Design review of the part built by this model. Coordinates are the model's own, in mm. Coordinates: 2 decimals unless noted, no trailing zeros. Write each loop counter-clockwise with the first axis right and the second up, starting at its lowest first coordinate (ties: lowest second). Pieces come first, ordered by that corner, then holes. Notation, with made-up numbers: M 60.25,-38.5 L 92.25,-38.5 A26 ccw 92.25,-21.5 Z; hole C -10.75,67.25 d7. An arc over 180 degrees is marked long. Write item = value, one per line.
```python
from build123d import *

# Parameters (mm, degrees)
BOSS_EXTRUDE1_DEPTH     = 5.5
CUT_EXTRUDE1_DEPTH      = 907.379197687
CUT_EXTRUDE1_DEPTH_BACK = 907.379197687
SKETCH2_R               = 1.6
SKETCH2_W               = 18
SKETCH2_H               = 13
SKETCH3_R               = 2.1
CUT_EXTRUDE2_DEPTH      = 907.379197687
SKETCH4_R               = 1.6
CUT_EXTRUDE3_DEPTH      = 907.379197687
SKETCH5_W               = 3.25
SKETCH5_H               = 9.45
SKETCH5_H_2             = 2.65
SKETCH5_W_2             = 1.25
SKETCH5_H_3             = 3.25
BOSS_EXTRUDE2_DEPTH     = 5.5


with BuildPart() as part:
    # Sketch1 → Boss-Extrude1 (new body)
    with BuildSketch(Plane.XY):
        Polygon((308.5, 78), (308.5, 50.625), (303, 50.625), (303, 42.125), (306.25, 42.125), (306.25, 40.5), (306.25, 38.875), (303, 38.875), (303, 30.375), (308.5, 30.375), (308.5, 3), (378, 3), (378, 8.5), (451.375, 8.5), (451.375, 17.95), (450.125, 17.95), (450.125, 20.6), (451.375, 20.6), (451.375, 23.25), (454.625, 23.25), (454.625, 20.6), (455.875, 20.6), (455.875, 17.95), (454.625, 17.95), (454.625, 8.5), (528, 8.5), (528, 3), (678, 3), (678, 8.5), (751.375, 8.5), (751.375, 17.95), (750.125, 17.95), (750.125, 20.6), (751.375, 20.6), (751.375, 23.25), (754.625, 23.25), (754.625, 20.6), (755.875, 20.6), (755.875, 17.95), (754.625, 17.95), (754.625, 8.5), (828, 8.5), (828, 3), (897.5, 3), (897.5, 30.375), (903, 30.375), (903, 38.875), (899.75, 38.875), (899.75, 40.5), (899.75, 42.125), (903, 42.125), (903, 50.625), (897.5, 50.625), (897.5, 78), align=None)
    extrude(amount=BOSS_EXTRUDE1_DEPTH)

    # Sketch2 → Cut-Extrude1 (cut, two sides: drawn at the far end of the back side and taken through both)
    with BuildSketch(Plane.XY.offset(5.5).offset(-CUT_EXTRUDE1_DEPTH_BACK)):
        with Locations((582.5, 40.5)):
            Circle(SKETCH2_R)
        with Locations((623.5, 40.5)):
            Circle(SKETCH2_R)
        with Locations((603, 40.5)):
            Rectangle(SKETCH2_W, SKETCH2_H)
    extrude(amount=CUT_EXTRUDE1_DEPTH + CUT_EXTRUDE1_DEPTH_BACK, mode=Mode.SUBTRACT)

    # Sketch3 → Cut-Extrude2 (cut, through all)
    with BuildSketch(Plane.XY.offset(5.5)):
        with Locations((503, 53)):
            Circle(SKETCH3_R)
        with Locations((503, 28)):
            Circle(SKETCH3_R)
        with Locations((703, 28)):
            Circle(SKETCH3_R)
        with Locations((703, 53)):
            Circle(SKETCH3_R)
    extrude(amount=-CUT_EXTRUDE2_DEPTH, mode=Mode.SUBTRACT)

    # Sketch4 → Cut-Extrude3 (cut, through all)
    with BuildSketch(Plane.XY.offset(5.5)):
        with Locations((343, 40.5)):
            Circle(SKETCH4_R)
        with Locations((863, 40.5)):
            Circle(SKETCH4_R)
    extrude(amount=-CUT_EXTRUDE3_DEPTH, mode=Mode.SUBTRACT)

    # Sketch5 → Boss-Extrude2 (add)
    with BuildSketch(Plane.XY.offset(5.5)):
        with Locations((753, 13.225)):
            Rectangle(SKETCH5_W, SKETCH5_H)
        with Locations((753, 19.275)):
            Rectangle(SKETCH5_W, SKETCH5_H_2)
        with Locations((750.75, 19.275)):
            Rectangle(SKETCH5_W_2, SKETCH5_H_2)
        with Locations((753, 21.925)):
            Rectangle(SKETCH5_W, SKETCH5_H_2)
        with Locations((755.25, 19.275)):
            Rectangle(SKETCH5_W_2, SKETCH5_H_2)
        with Locations((901.375, 40.5)):
            Rectangle(SKETCH5_W, SKETCH5_H_3)
        with Locations((453, 13.225)):
            Rectangle(SKETCH5_W, SKETCH5_H)
        with Locations((453, 19.275)):
            Rectangle(SKETCH5_W, SKETCH5_H_2)
        with Locations((453, 21.925)):
            Rectangle(SKETCH5_W, SKETCH5_H_2)
        with Locations((450.75, 19.275)):
            Rectangle(SKETCH5_W_2, SKETCH5_H_2)
        with Locations((455.25, 19.275)):
            Rectangle(SKETCH5_W_2, SKETCH5_H_2)
        with Locations((304.625, 40.5)):
            Rectangle(SKETCH5_W, SKETCH5_H_3)
    extrude(amount=-BOSS_EXTRUDE2_DEPTH)


solid = part.part
```
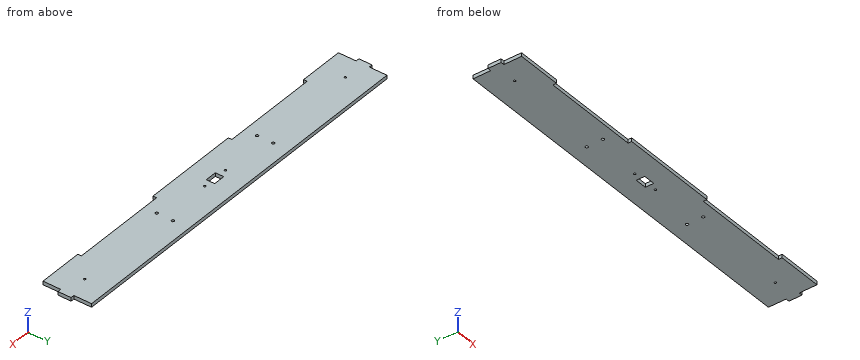
Q1. Consider section B-B, the plane z = 3.7. State how many separate pieces and enclosed holes the cut face has, and give its area (3 significant figures).
Check result:
separate_pieces = 1
enclosed_holes = 9
area = 42,400 mm²
Q2. Wall thickness on line 1 (Y direction, x = 503, z = 1.9); line 2 (X direction, y = 42.5, z = 4.1); line 3 (Y direction, x = 582.5, z = 2.6): over which ranges is each line inside the solid? List them lowest first.
Check result:
line_1 = 8.5 to 25.9, 30.1 to 50.9, 55.1 to 78
line_2 = 303 to 594, 612 to 903
line_3 = 3 to 38.9, 42.1 to 78
Q3. Consider section A-A, the plane x = 604.5. State the section outline as (y, z) points, and give its area (3 significant figures).
Check result:
outline = M 3,0 L 34,0 L 34,5.5 L 3,5.5 Z; M 47,0 L 78,0 L 78,5.5 L 47,5.5 Z
area = 341 mm²
Q4. For P1, Ø3, axis at x = 901, z = 2, coming from the +Y side (3 decimals); P2, Ø3, axis at y = 60, z = 2, coming from the +X side; P3, Ø2.5, axis at x = 503, y = 53, coming from the +Z side; P4, Ø1.6, axis at y = 18.5, z = 2, coming from the -X side, all flat-tipped, find the tip position at first contact; note any pin that passes through.
Check result:
P1 = 50.625
P2 = 897.5
P3 = through
P4 = 308.5
Q5. Consider section C-C, the plane x = 811.5. State the section outline as (y, z) points, and give its area (3 significant figures).
Check result:
outline = M 8.5,0 L 78,0 L 78,5.5 L 8.5,5.5 Z
area = 382 mm²
